```python
from build123d import *

# Parameters (mm, degrees)
SKETCH_1_R      = 6.5
EXTRUDE_1_DEPTH = 8


with BuildPart() as part:
    # Эскиз1 → Бобышка-Вытянуть1 (new body)
    with BuildSketch(Plane.XZ):
        with BuildLine():
            Line((7.24137931, -6.896551724), (9.113300493, -4.931034483))
            ThreePointArc((9.113300493, -4.931034483), (10.10395639, -4.24256491), (11.285714286, -4))
            Line((11.285714286, -4), (238.714285714, -4))
            ThreePointArc((238.714285714, -4), (239.89604361, -4.24256491), (240.886699507, -4.931034483))
            Line((240.886699507, -4.931034483), (242.75862069, -6.896551724))
            ThreePointArc((242.75862069, -6.896551724), (260, 0), (242.75862069, 6.896551724))
            Line((242.75862069, 6.896551724), (240.886699507, 4.931034483))
            ThreePointArc((240.886699507, 4.931034483), (239.89604361, 4.24256491), (238.714285714, 4))
            Line((238.714285714, 4), (11.285714286, 4))
            ThreePointArc((11.285714286, 4), (10.10395639, 4.24256491), (9.113300493, 4.931034483))
            Line((9.113300493, 4.931034483), (7.24137931, 6.896551724))
            ThreePointArc((7.24137931, 6.896551724), (-10, 0), (7.24137931, -6.896551724))
        make_face()
        with Locations(Location((0, 0, 0), (0, 0, 90))):
            Circle(SKETCH_1_R, mode=Mode.SUBTRACT)
        with Locations(Location((250, 0, 0), (0, 0, 90))):
            Circle(SKETCH_1_R, mode=Mode.SUBTRACT)
    extrude(amount=-EXTRUDE_1_DEPTH)


solid = part.part
```
Design review of the part built by this model. Coordinates are the model's own, in mm. A direction names the side the tool comes from. Give positions to 0.01 mm unless a question says otherwise; leave off trailing zeros. Write each loop counter-clockwise with the first axis right and the second up, starting at its lowest first coordinate (ties: lowest second). Pieces come first, ordered by that corner, then holes. Notation, with made-up numbers: (51, -35.75) - (82, -35.75) arc R20 cw to (82, -4.75) - close; hole circle Ø8 at (10, 89.25). An arc over 180 degrees is marked (long way). Return JSON: item names as keys, results as strings. Group by question number.
(1) To check wall thickness, follow probe 1 along X at (y, z) = (5.75, 0); probe 2 along X at (y, z) = (2.25, -5.5); probe 3 along X at (y, z) = (7.5, -4.5). State the ranges of each line that lie inside material, in increasing order.
(2) We need section B-B, the plane x = 0. Give the boundary of the cut face in (y, z).
(3) Insertion check: pin 1 (4 mm diameter, centred on x = 231.5, y = 5, fed in from -Z); pin 2 (1 mm diameter, centred on y = 4.5, z = -3.5, fed in from +X). Each pin has a flat end and moves straight along its axis. Give the tip position at first contact, or say it passes through.
(4) We need section D-D, the plane x = 183.5. Give the boundary of the cut face in (y, z).
(5) Machinability: for faces 3 (the flat face through (127, 4, 4)), 4 (the cylindrical face through (255.767, 3.944, 2.999)), 5 (the flat face through (123, 4, -4)), which of the approach directions +Z, -Z, +X, -X, +Y, -Y give a long, thin tool a straight path to every point of the face, cutting with its end or side? Answer none if there is none.
(6) We need section C-C, the plane y = 1.25. Give the boundary of the cut face in (x, z), then the cut area to 3 significant figures.
(7) We need section A-A, the plane z = 0. Give the boundary of the cut face in (x, y).
(8) Mouldability with a two-part tool opening along X and no side actions: class faces 1 (the cylindrical face through (3.955, 3.944, -5.158)), 2 (the flat face through (123, 8, 0)) as +X half, -X half, draft (parallel to the pull), parting line (faces both ways), or undercut.
Reported:
{
 "1": {"probe 1": "x = -10 to -6.5, 6.5 to 243.5, 256.5 to 260", "probe 2": "x = -8.35 to -3.46, 3.46 to 8.57, 241.43 to 246.54, 253.46 to 258.35", "probe 3": "x = -8.93 to -4.69, 4.69 to 9.63, 240.37 to 245.31, 254.69 to 258.93"},
 "2": {"outline": "(0, -10) - (8, -10) - (8, -6.5) - (0, -6.5) - close; (0, 6.5) - (8, 6.5) - (8, 10) - (0, 10) - close"},
 "3": {"pin 1": "stops at z = -4", "pin 2": "stops at x = 259.54"},
 "4": {"outline": "(0, -4) - (8, -4) - (8, 4) - (0, 4) - close"},
 "5": {"face 3": "+Z, +Y, -Y", "face 4": "+Y, -Y", "face 5": "-Z, +Y, -Y"},
 "6": {"outline": "(7.24, -6.9) - (9.11, -4.93) arc R3 cw to (11.29, -4) - (238.71, -4) arc R3 cw to (240.89, -4.93) - (242.76, -6.9) arc R10 ccw (long way) to (242.76, 6.9) - (240.89, 4.93) arc R3 cw to (238.71, 4) - (11.29, 4) arc R3 cw to (9.11, 4.93) - (7.24, 6.9) arc R10 ccw (long way) to start; hole circle Ø13 at (0, 0); hole circle Ø13 at (250, 0)", "area": "2,210 mm2"},
 "7": {"outline": "(-10, 0) - (-6.5, 0) - (-6.5, 8) - (-10, 8) - close; (6.5, 0) - (243.5, 0) - (243.5, 8) - (6.5, 8) - close; (256.5, 0) - (260, 0) - (260, 8) - (256.5, 8) - close"},
 "8": {"face 1": "undercut", "face 2": "draft"}
}
